The model under review builds one solid part; all positions refer to its coordinate system, in mm. A direction names the side the tool comes from. Coordinates: 2 decimals unless noted, no trailing zeros. Loops run counter-clockwise (first coordinate to the right, second up) from the corner with the lowest first, then second, coordinate; pieces in that order, holes last. Notation, with made-up numbers: M 16.5,-20 L 25.5,-20 A21 ccw 25.5,15 Z; hole C -27,38.5 d3. An arc over 180 degrees is marked long. Use CSV: the item, a comma, the result in double quotes. Start each with the question number.
1. Tool access review of faces 1 (the flat face through (-3.4, -3, 0)), 2 (the cylindrical face through (-13.77, -61.99, 18.96)): name each direction out of +Z, -Z, +X, -X, +Y, -Y from which nothing blocks a thin tool from reaching the whole face with its end or side.
2. Clearance check with flat-ended pins moving along their axes: P1, Ø12, axis at y = -17, z = 18.5, coming from the -X side; P2, Ø1.5, axis at y = -3, z = 3, coming from the -X side; P3, Ø4, axis at x = 11, z = 9.5, coming from the +Y side. State where each tip first meets the part, or that it passes through.
3. Add section A-A, the plane x = 0. Write out the cut boundary in (y, z), then the cut area to 3 significant figures.
4. Add section C-C, the plane z = -2.25. Write out the cut boundary in (x, y), then the cut area to 3 significant figures.
5. Add section D-D, the plane z = 9. Write out the cut boundary in (x, y), then the cut area to 3 significant figures.
6. For L1, parallel to Z at x = 45.5, y = 14; L2, parallel to Y at x = 15, z = 17.25; L3, parallel to X at y = -9, z = 12, list the stretches that pass through material, from the lowest coordinate up.
from build123d import *

# Parameters (mm, degrees)
F0_R     = 14.25
F0_R_2   = 2.5
F1_DEPTH = 16
F2_DEPTH = 19
F3_R     = 63.5
F4_DEPTH = 6
F5_R     = 4.15
F6_DEPTH = 4


with BuildPart() as f1:
    # F0 (on Top) → F1 (new body)
    with BuildSketch(Plane.XY):
        Circle(F0_R)
        Circle(F0_R_2, mode=Mode.SUBTRACT)
    extrude(amount=F1_DEPTH)

    # F0 (on Top) → F2 (join)
    with BuildSketch(Plane.XY):
        Circle(F0_R_2)
    extrude(amount=F2_DEPTH)

    # F3 (on face) → F4 (join)
    with BuildSketch(Plane.XY.offset(16)):
        Circle(F3_R)
    extrude(amount=F4_DEPTH)

    # F5 (on face) → F6 (join)
    with BuildSketch(Plane(origin=(0, 0, 0), x_dir=(1, 0, 0), z_dir=(0, 0, -1))):
        Circle(F5_R)
    extrude(amount=F6_DEPTH)


solid = f1.part
Computed:
1,face 1,"-Z"
1,face 2,"+Z, -Z"
2,P1,"stops at x = -62.54"
2,P2,"stops at x = -14.07"
2,P3,"stops at y = 11.05"
3,outline,"M -63.5,16 L -14.25,16 L -14.25,0 L -4.15,0 L -4.15,-4 L 4.15,-4 L 4.15,0 L 14.25,0 L 14.25,16 L 63.5,16 L 63.5,22 L -63.5,22 Z"
3,area,"1,250 mm^2"
4,outline,"C 0,0 d8.3"
4,area,"54.1 mm^2"
5,outline,"C 0,0 d28.5"
5,area,"638 mm^2"
6,L1,"z = 16 to 22"
6,L2,"y = -61.7 to 61.7"
6,L3,"x = -11.05 to 11.05"
